The listing builds one solid part. Answer for the finished solid, in the listing's coordinates (mm). A direction names the side the tool comes from. Round coordinates to 2 decimals unless told otherwise and drop trailing zeros. Loops run counter-clockwise (first coordinate to the right, second up) from the corner with the lowest first, then second, coordinate; pieces in that order, holes last. Notation, with made-up numbers: (19, 46.5) - (51, 46.5) arc R17 ccw to (51, 76.5) - close; hole circle Ø7 at (52.5, 87). An arc over 180 degrees is marked (long way). One line per item, written item: value.
```python
from build123d import *

# Parameters (mm, degrees)
BOSS_EXTRUDE1_DEPTH = 60
BOSS_EXTRUDE2_DEPTH = 2
FILLET1_R           = 0.5


with BuildPart() as part:
    # Sketch2 → Boss-Extrude1 (new body)
    with BuildSketch(Plane(origin=(0, 0, 0), x_dir=(1, 0, 0), z_dir=(0, 1, 0))):
        Polygon((-20.575, 0), (20.575, 0), (20.575, 2.4), (17.825, 2.4), (8.5, 9.4), (8.5, 11.805044241), (10.5, 11.805044241), (10.5, 10.399464037), (18.492143163, 4.4), (22.575, 4.4), (22.575, -2), (-22.575, -2), (-22.575, 4.4), (-18.492143163, 4.4), (-10.5, 10.399464037), (-10.5, 11.805044241), (-8.5, 11.805044241), (-8.5, 9.4), (-17.825, 2.4), (-20.575, 2.4), align=None)
    extrude(amount=BOSS_EXTRUDE1_DEPTH)

    # Sketch4 → Boss-Extrude2 (add)
    with BuildSketch(Plane(origin=(0, 60, 0), x_dir=(1, 0, 0), z_dir=(0, 1, 0))):
        Polygon((-22.575, 4.4), (-22.575, -2), (22.575, -2), (22.575, 4.4), (18.492143163, 4.4), (10.5, 10.399464037), (10.5, 11.805044241), (-10.5, 11.805044241), (-10.5, 10.399464037), (-18.492143163, 4.4), align=None)
    extrude(amount=BOSS_EXTRUDE2_DEPTH)

    # Fillet1
    fillet1_edges = [part.edges().sort_by_distance(p)[0] for p in [
        (8.5, 30, -9.4),
        (18.492143163, 31, -4.4),
        (22.575, 31, -4.4),
        (22.575, 31, 2),
        (-22.575, 31, 2),
        (-22.575, 31, -4.4),
        (-18.492143163, 31, -4.4),
        (-8.5, 30, -9.4),
        (-20.575, 30, -2.4),
        (-20.575, 30, 0),
        (20.575, 30, 0),
        (20.575, 30, -2.4),
    ]]
    fillet(fillet1_edges, radius=FILLET1_R)


solid = part.part
```
1) A cutting plane is placed at D-D on x = 17. Give the vertices of the cut face in (y, z).
Final values:
outline: (0, -5.52) - (62, -5.52) - (62, 2) - (0, 2) - (0, 0) - (60, 0) - (60, -3.02) - (0, -3.02) - close
2) For faces 1 (the flat face through (-10.5, 31, -11)), 2 (the flat face through (10.5, 31, -11)), 3 (the flat face through (0, 62, -3)), 4 (the flat face through (13.326, 29.58, -5.777)), determine the directions among +Z, -Z, +X, -X, +Y, -Y from which every point of the face is accessible in a straight line to the end or side of a thin tool.
Final values:
face 1: -Z, -X, +Y, -Y
face 2: -Z, +X, +Y, -Y
face 3: +Z, -Z, +X, -X, +Y
face 4: -Y
3) Each of these flat-tipped pins is pushed along its axis until it touches: pin 1 Ø1.7 at (x, y) = (20.5, 29) entering from -Z; pin 2 Ø6 at (x, z) = (1.5, -4.5) entering from -Y; pin 3 Ø1.5 at (y, z) = (44, -11) entering from -X. Where does it stop, or does it pass through?
Final values:
pin 1: z = -4.4
pin 2: y = 60
pin 3: x = -10.7
4) Consider L1, parallel to Z at x = 20, y = 44; L2, parallel to X at y = 40.5, z = -10.5; L3, parallel to X at y = 7, z = -0.75 (3 decimals). Determine where each line is inside the solid, lowest interval first.
Final values:
L1: -4.4 to -2.4, 0 to 2
L2: -10.5 to -8.5, 8.5 to 10.5
L3: -22.575 to -20.575, 20.575 to 22.575
5) For a pull along Z with two mould halves and no side action, classify faces 5 (the flat face through (-14.374, 30.566, -7.491)), 6 (the flat face through (-8.5, 30, -11)), 7 (the flat face through (-19, 30, -2.4)), 8 (the flat face through (0, 31, 2)) as released by +Z, released by -Z, zero draft, split by the parting line, or undercut.
Final values:
face 5: released by -Z
face 6: zero draft
face 7: undercut
face 8: released by +Z
6) A cutting plane is placed at C-C on z = -6. Give the vertices of the cut face in (x, y).
Final values:
outline: (-16.36, 0) - (-13.03, 0) - (-13.03, 60) - (13.03, 60) - (13.03, 0) - (16.36, 0) - (16.36, 62) - (-16.36, 62) - close
7) A cutting plane is placed at A-A on x = 6.5. Give the vertices of the cut face in (y, z).
Final values:
outline: (0, 0) - (60, 0) - (60, -11.81) - (62, -11.81) - (62, 2) - (0, 2) - close
